For this review, use the dimensioned drawing (mm, ordinates from the lowest corner) and the shaded views. A direction names the side the tool comes from. Give positions to 0.01 mm unless a question says otherwise; leave off trailing zeros. Loops run counter-clockwise (first coordinate to the right, second up) from the corner with the lowest first, then second, coordinate; pieces in that order, holes last. Notation, with made-up numbers: (59.25, -21.5) -> (99.25, -21.5) arc R23 cw to (99.25, 2.5) -> close; hole circle Ø7 at (-2.5, 9.25). An arc over 180 degrees is marked (long way). Write each question's results on one line, items separated by ' | '. Start each with the question number.
Q1. We need section A-A (z = 3.65). Write out the cut boundary in (x, y).
Q2. Insertion check: pin 1 Ø2 at (x, z) = (3.5, 2.5) entering from +Y; pin 2 Ø1.9 at (y, z) = (20.5, 4) entering from -X. Each pin has a flat end and moves straight along its axis. Give the tip position at first contact, or say it passes through.
Q3. Mouldability with a two-part tool opening along Y and no side actions: class the marked faces 1, 2 and 3 as released by +Y, released by -Y, zero draft, split by the parting line, or undercut.
Q4. We need section C-C (y = 5). Write out the cut boundary in (x, z).
Q5. Wall thickness on L1, parallel to Z at x = 11.75, y = 8.5; L2, parallel to X at y = 18.75, z = 5.75; L3, parallel to Y at x = 8, z = 5.5: over which ranges is each line inside the solid? List them lowest first. Write a range as [from, to].
Q6. We need section B-B (x = 8). Write out the cut boundary in (y, z), plus the area to 3 significant figures.
Q7. Machinability: for the marked faces 4, 5, 6, 7 and 8, which of the approach directions +Z, -Z, +X, -X, +Y, -Y give a long, thin tool a straight path to every point of the face, cutting with its end or side? Answer none if there is none.
Q8. We need section D-D (z = 1.5). Write out the cut boundary in (x, y).
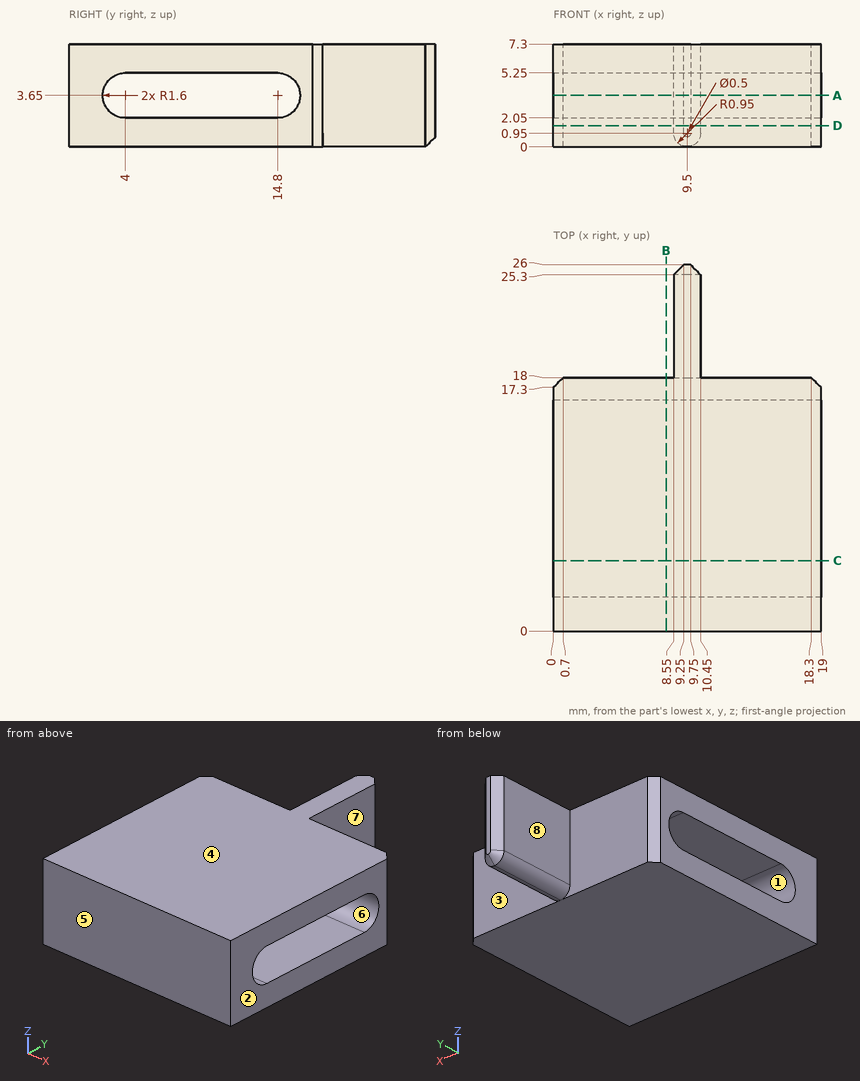
Output:
1) outline: (0, 0) -> (19, 0) -> (19, 2.4) -> (0, 2.4) -> close; (0, 16.4) -> (19, 16.4) -> (19, 17.3) -> (18.3, 18) -> (10.45, 18) -> (10.45, 25.3) -> (9.75, 26) -> (9.25, 26) -> (8.55, 25.3) -> (8.55, 18) -> (0.7, 18) -> (0, 17.3) -> close
2) pin 1: y = 18 | pin 2: x = 8.55
3) face 1: undercut | face 2: zero draft | face 3: released by +Y
4) outline: (0, 0) -> (19, 0) -> (19, 2.05) -> (0, 2.05) -> close; (0, 5.25) -> (19, 5.25) -> (19, 7.3) -> (0, 7.3) -> close
5) L1: [0, 2.05], [5.25, 7.3] | L2: [8.55, 10.45] | L3: [0, 18]
6) outline: (0, 0) -> (18, 0) -> (18, 7.3) -> (0, 7.3) -> close; hole (4, 2.05) -> (14.8, 2.05) arc R1.6 ccw to (14.8, 5.25) -> (4, 5.25) arc R1.6 ccw to start | area: 88.8 mm2
7) face 4: +Z, +X, -X, +Y, -Y | face 5: +Z, -Z, +X, -X, -Y | face 6: +X, -X | face 7: +Z, -Z, +X, +Y | face 8: +Z, -Z, -X, +Y
8) outline: (0, 0) -> (19, 0) -> (19, 17.3) -> (18.3, 18) -> (10.45, 18) -> (10.45, 25.3) -> (9.75, 26) -> (9.25, 26) -> (8.55, 25.3) -> (8.55, 18) -> (0.7, 18) -> (0, 17.3) -> close
